Work out the finished part from the listing and answer in its coordinate system (mm). A direction names the side the tool comes from. Give positions to 0.01 mm unless a question says otherwise; leave off trailing zeros. Write each loop counter-clockwise with the first axis right and the second up, starting at its lowest first coordinate (ties: lowest second). Pieces come first, ordered by that corner, then holes. Notation, with made-up numbers: (-28.75, 40.5) -> (29.25, 40.5) arc R6 ccw to (29.25, 51.5) -> close; hole circle Ø9 at (57.25, 43.25). An arc over 180 degrees is marked (long way). Use a Markdown table: item, result. Add a question column.
Q1. Section B-B, the plane y = -43 is taken. Give the vertices of the cut face in (x, z), plus the area to 3 significant figures.
Q2. Section A-A, the plane x = 14 is taken. Give the vertices of the cut face in (y, z), plus the area to 3 significant figures.
Q3. Section C-C, the plane x = 22 is taken. Give the vertices of the cut face in (y, z).
Q4. Each of these flat-tipped pins is pushed along its axis until it touches: pin 1 Ø2 at (x, z) = (6, 1) entering from +Y; pin 2 Ø3 at (y, z) = (1, 4) entering from -X; pin 3 Ø3 at (x, y) = (30, -39.5) entering from +Z. Where does it stop, or does it pass through?
Q5. Consider line 1 (Z direction, x = 24, y = -25); line 2 (Y direction, x = 6, z = 1.5); line 3 (Y direction, x = 22, z = 4). Determine where each line is inside the solid, lowest interval first.
Q6. For faces 1 (the face through (10, 0, 1)), 2 (the face through (40, -30, 1)), determine the directions among +Z, -Z, +X, -X, +Y, -Y from which every point of the face is accessible in a straight line to the end or side of a thin tool.
from build123d import *

# Parameters (mm, degrees)
F0_W     = 40
F0_H     = 81
F1_DEPTH = 1.8
F3_DEPTH = 20


with BuildPart() as f1:
    # F0 (on Top) → F1 (new body)
    with BuildSketch(Plane.XY):
        with Locations((20, -40.5)):
            Rectangle(F0_W, F0_H)
    extrude(amount=F1_DEPTH)

    # F2 (on face) → F3 (join)
    with BuildSketch(Plane.YZ.offset(40)):
        with BuildLine():
            Line((0, 1.8), (0, 0))
            ThreePointArc((0, 0), (2.1213203436, 0.8786796564), (3, 3))
            ThreePointArc((3, 3), (-0.6129289311, 5.9367189388), (-2.749545417, 1.8))
            Line((-2.749545417, 1.8), (0, 1.8))
        make_face()
        with BuildLine():
            ThreePointArc((-2.749545417, 1.8), (-1.6431676725, 0.4900199204), (0, 0))
            Line((0, 0), (0, 1.8))
            Line((0, 1.8), (-2.749545417, 1.8))
        make_face()
    extrude(amount=-F3_DEPTH)


solid = f1.part
Result set:
| question | item | result |
|---|---|---|
| 1 | outline | (0, 0) -> (40, 0) -> (40, 1.8) -> (0, 1.8) -> close |
| 1 | area | 72.0 mm2 |
| 2 | outline | (-81, 0) -> (0, 0) -> (0, 1.8) -> (-81, 1.8) -> close |
| 2 | area | 146 mm2 |
| 3 | outline | (-81, 0) -> (0, 0) arc R3 ccw (long way) to (-2.75, 1.8) -> (-81, 1.8) -> close |
| 4 | pin 1 | stops at y = 0 |
| 4 | pin 2 | stops at x = 20 |
| 4 | pin 3 | stops at z = 1.8 |
| 5 | line 1 | z = 0 to 1.8 |
| 5 | line 2 | y = -81 to 0 |
| 5 | line 3 | y = -2.83 to 2.83 |
| 6 | face 1 | +Z, -Z, -X, +Y |
| 6 | face 2 | +Z, -Z, +X, +Y, -Y |
